Model file for the job. Use its own axes, mm. A direction names the side the tool comes from. Round coordinates to 2 decimals unless told otherwise and drop trailing zeros. Loops run counter-clockwise (first coordinate to the right, second up) from the corner with the lowest first, then second, coordinate; pieces in that order, holes last. Notation, with made-up numbers: (63, 61) - (67, 61) arc R21 ccw to (67, 100) - close; hole circle Ø9 at (82, 63.5). An arc over 180 degrees is marked (long way). Answer as a JSON object with one key per item and string values.
from build123d import *

# Parameters (mm, degrees)
F1_DEPTH    = 5
F3_W        = 10
F3_H        = 180
F4_DEPTH    = 5.001
F5_T1_DEPTH = 146.7820454904
F6_R        = 2
F11_DEPTH   = 25
F13_DEPTH   = 25
F14_R       = 2


# Not quite as in the source:
# - a fillet or chamfer that OpenCascade refuses, or shapes differently, is made with other operations: its cross-section is extruded or revolved along the edge and cut away or added
# - two fillets or chamfers of one size are made in one step


with BuildPart() as f1:
    # F0 (on Front) → F1 (new body)
    with BuildSketch(Plane.XZ):
        Polygon((-46.3970234266, 0), (0, 0), (0, 8), (-5, 8), (-5, 5), (-10, 5), (-46.3970234266, 105), align=None)
        Polygon((-41.3970234266, 5), (-41.3970234266, 76.6435909019), (-15.3208888624, 5), align=None, mode=Mode.SUBTRACT)
    extrude(amount=-F1_DEPTH)

    # F3 (on face) → F4 (cut, through all)
    with BuildSketch(Plane.XY.offset(5)):
        with Locations((-5, 95)):
            Rectangle(F3_W, F3_H)
    extrude(amount=-F4_DEPTH, mode=Mode.SUBTRACT)

    # F5: fillet of radius 5 on 1 edges, made by hand

    # F5_s2 → F5_t1 (cut)
    with BuildSketch(Plane.XZ.offset(-75.8910227452)):
        with BuildLine():
            ThreePointArc((-46.3970234266, 76.6435909019), (-42.265264315, 81.567629667), (-36.6985603227, 78.3536916185))
            Line((-36.6985603227, 78.3536916185), (-46.3970234266, 105))
            Line((-46.3970234266, 105), (-46.3970234266, 76.6435909019))
        make_face()
    extrude(amount=F5_T1_DEPTH, mode=Mode.SUBTRACT)

    # F6
    f6_edges = [f1.edges().sort_by_distance(p)[0] for p in [
        (-46.397023, 0, 38.321795),
        (-46.397023, 5, 38.321795),
        (-42.265264, 0, 81.56763),
        (-23.34928, 0, 41.676846),
        (-7.5, 0, 5),
        (-5, 0, 6.5),
        (-2.5, 0, 8),
        (0, 0, 4),
        (-28.358956, 0, 5),
        (-7.5, 5, 5),
        (-5, 5, 6.5),
        (-2.5, 5, 8),
        (0, 5, 4),
        (-42.265264, 5, 81.56763),
        (-23.34928, 5, 41.676846),
        (-28.358956, 5, 5),
        (-5, 2.5, 8),
        (0, 2.5, 8),
    ]]
    fillet(f6_edges, radius=F6_R)

    # F10 (on face) → F11 (join)
    with BuildSketch(Plane.XZ):
        Polygon((-44.3970234266, 3), (-44.3970234266, 0), (-27.9949859102, 0), (-27.9949859102, 3), (-41.3970234266, 3), align=None)
    extrude(amount=F11_DEPTH)

    # F12 (on face) → F13 (join)
    with BuildSketch(Plane(origin=(0, 5, 0), x_dir=(-1, 0, 0), z_dir=(0, 1, 0))):
        Polygon((27.9949859102, 0), (44.3970234266, 0), (44.3970234266, 3), (41.3970234266, 3), (27.9949859102, 3), align=None)
    extrude(amount=F13_DEPTH)

    # F14
    f14_edges = [f1.edges().sort_by_distance(p)[0] for p in [
        (-27.994986, -25, 1.5),
        (-44.397023, -25, 1.5),
        (-36.196005, -25, 3),
        (-27.994986, -12.5, 3),
        (-44.397023, -12.5, 3),
        (-27.994986, 30, 1.5),
        (-44.397023, 30, 1.5),
        (-27.994986, 17.5, 3),
        (-36.196005, 30, 3),
        (-44.397023, 17.5, 3),
    ]]
    fillet(f14_edges, radius=F14_R)


solid = f1.part
1) Tool access for faces 1 (the cylindrical face through (-28.18, 4.43, 4.4)), 2 (the cylindrical face through (-43.827, 16.661, 2.399)), 3 (the cylindrical face through (-7.26, 4.65, 4.13)): list every direction of +Z, -Z, +X, -X, +Y, -Y with a clear straight run to the whole face (end or side of a thin tool).
Values follow:
{"face 1": "+Y", "face 2": "+Z, -X, +Y", "face 3": "+Z, +Y"}
2) Slice it at A-A on x = -7.5. List the corners of the cut face in (y, z).
Values follow:
{"outline": "(0, 0) - (5, 0) - (5, 3) arc R2 ccw to (3, 5) - (2, 5) arc R2 ccw to (0, 3) - close"}
3) Slice it at B-B on y = 21. List the corners of the cut face in (x, z), then the cut area to 3 significant figures.
Values follow:
{"outline": "(-44.4, 0) - (-27.99, 0) - (-27.99, 1) arc R2 ccw to (-29.99, 3) - (-42.4, 3) arc R2 ccw to (-44.4, 1) - close", "area": "47.5 mm²"}
4) Two-plate mould, pull along X, no slides. Class faces 4 (the cylindrical face through (-4.13, 4.65, 5.15)), 5 (the cylindrical face through (-0.6, 4.43, 3.04)), 6 (the cylindrical face through (-36.28, -24.43, 2.4)): pulls with the +X half, pulls with the -X half, needs draft (parallel to the pull), parting line crosses it, or undercut.
Values follow:
{"face 4": "undercut", "face 5": "pulls with the +X half", "face 6": "needs draft"}
5) Probe probe 1 along X at (y, z) = (4, 17); probe 2 along X at (y, z) = (0.5, 21.5); probe 3 along Y at (x, z) = (-23.5, 36). List the from-to ranges inside material, lowest first.
Values follow:
{"probe 1": "-46.13 to -41.4, -19.69 to -14.65", "probe 2": "-45.72 to -41.4, -21.33 to -16.73", "probe 3": "0 to 5"}
6) Drop flat-ended pins along their axis: P1, Ø0.5, axis at y = -10.5, z = 0.5, coming from the +X side (3 decimals); P2, Ø1.1, axis at x = -8, y = 2.5, coming from the +Z side; P3, Ø3, axis at x = -15, z = 18.5, coming from the -Y side. Give the stop position or say it passes through.
Values follow:
{"P1": "x = -27.995", "P2": "z = 5", "P3": "y = 0.04"}
